Build history of the part. All positions in model axes, mm. Give positions to 0.01 mm unless a question says otherwise; leave off trailing zeros. Order: outer loops, then holes, each group sorted by start corner. A loop starts at its lowest first (then second) coordinate and runs counter-clockwise, first axis right, second up. Notation, with made-up numbers: (33.5, -39.75) - (59.5, -39.75) arc R21 ccw to (59.5, -26.75) - close; hole circle Ø6 at (-20, 63.25). An arc over 180 degrees is marked (long way). Answer in a Markdown table with one row per item.
```python
from build123d import *

# Parameters (mm, degrees)
F0_R     = 1.25
F0_R_2   = 5.5
F1_DEPTH = 4
F3_DEPTH = 2
F4_SIZE  = 2


# Not quite as in the source:
# - a feature names something its author has since deleted; it is built from what else it names


with BuildPart() as f1:
    # F0 (on Top) → F1 (new body)
    with BuildSketch(Plane.XY):
        with BuildLine():
            ThreePointArc((-36.0336562554, 5.4360876058), (-41.0336562554, 10.4360876058), (-46.0336562554, 5.4360876058))
            ThreePointArc((-46.0336562554, 5.4360876058), (-48.7113140605, 0.9910484741), (-53.6336562554, -0.6517453414))
            Line((-53.6336562554, -0.6517453414), (-57.6336562554, -0.6517453414))
            Line((-57.6336562554, -0.6517453414), (-59.4336562554, -0.6517453414))
            Line((-59.4336562554, -0.6517453414), (-59.4336562554, -1.3484233022))
            ThreePointArc((-59.4336562554, -1.3484233022), (-52.8307134237, -18.2761605269), (-36.5097932518, -26.2620672584))
            Line((-36.5097932518, -26.2620672584), (33.4902067482, -32.0954005917))
            ThreePointArc((33.4902067482, -32.0954005917), (52.4940809692, -25.5788138039), (60.5663437446, -7.1817566356))
            Line((60.5663437446, -7.1817566356), (60.5663437446, 8.4782659528))
            ThreePointArc((60.5663437446, 8.4782659528), (52.4940809692, 26.8753231211), (33.4902067482, 33.3919099089))
            Line((33.4902067482, 33.3919099089), (-36.5097932518, 27.5585765756))
            ThreePointArc((-36.5097932518, 27.5585765756), (-52.8307134237, 19.5726698441), (-59.4336562554, 2.6449326195))
            Line((-59.4336562554, 2.6449326195), (-59.4336562554, 1.9482546586))
            Line((-59.4336562554, 1.9482546586), (-57.6336562554, 1.9482546586))
            Line((-57.6336562554, 1.9482546586), (-53.6336562554, 1.9482546586))
            ThreePointArc((-53.6336562554, 1.9482546586), (-50.3543429782, 2.8450290737), (-48.4065189788, 5.6314392355))
            ThreePointArc((-48.4065189788, 5.6314392355), (-40.8279863477, 12.5929298404), (-33.4336562554, 5.4360876058))
            ThreePointArc((-33.4336562554, 5.4360876058), (-31.5267024615, 2.8420068396), (-28.4336562554, 1.9482546586))
            Line((-28.4336562554, 1.9482546586), (-15.4336562554, 1.9482546586))
            Line((-15.4336562554, 1.9482546586), (-15.4336562554, 15.2482546586))
            Line((-15.4336562554, 15.2482546586), (-4.9336562554, 15.2482546586))
            Line((-4.9336562554, 15.2482546586), (-4.9336562554, 17.1757546586))
            ThreePointArc((-4.9336562554, 17.1757546586), (-0.8336562554, 21.2757546586), (3.2663437446, 17.1757546586))
            Line((3.2663437446, 17.1757546586), (3.2663437446, 15.2482546586))
            Line((3.2663437446, 15.2482546586), (29.2163437446, 15.2482546586))
            Line((29.2163437446, 15.2482546586), (29.2163437446, 17.1757546586))
            ThreePointArc((29.2163437446, 17.1757546586), (33.3163437446, 21.2757546586), (37.4163437446, 17.1757546586))
            Line((37.4163437446, 17.1757546586), (37.4163437446, 15.2482546586))
            Line((37.4163437446, 15.2482546586), (47.9163437446, 15.2482546586))
            Line((47.9163437446, 15.2482546586), (47.9163437446, -13.9517453414))
            Line((47.9163437446, -13.9517453414), (37.4163437446, -13.9517453414))
            Line((37.4163437446, -13.9517453414), (37.4163437446, -15.8792453414))
            ThreePointArc((37.4163437446, -15.8792453414), (33.3163437446, -19.9792453414), (29.2163437446, -15.8792453414))
            Line((29.2163437446, -15.8792453414), (29.2163437446, -13.9517453414))
            Line((29.2163437446, -13.9517453414), (3.2663437446, -13.9517453414))
            Line((3.2663437446, -13.9517453414), (3.2663437446, -15.8792453414))
            ThreePointArc((3.2663437446, -15.8792453414), (-0.8336562554, -19.9792453414), (-4.9336562554, -15.8792453414))
            Line((-4.9336562554, -15.8792453414), (-4.9336562554, -13.9517453414))
            Line((-4.9336562554, -13.9517453414), (-15.4336562554, -13.9517453414))
            Line((-15.4336562554, -13.9517453414), (-15.4336562554, -0.6517453414))
            Line((-15.4336562554, -0.6517453414), (-28.4336562554, -0.6517453414))
            ThreePointArc((-28.4336562554, -0.6517453414), (-33.3559984503, 0.991048474), (-36.0336562554, 5.4360876058))
        make_face()
        with Locations((-34.4336562554, -13.8484233022)):
            Circle(F0_R, mode=Mode.SUBTRACT)
        with Locations((33.4902067482, -25.3792453414)):
            Circle(F0_R, mode=Mode.SUBTRACT)
        with Locations((-34.4336562554, 15.1449326195)):
            Circle(F0_R, mode=Mode.SUBTRACT)
        with Locations((33.4321971192, 26.6757546586)):
            Circle(F0_R, mode=Mode.SUBTRACT)
        with BuildLine():
            ThreePointArc((-53.6336562554, -0.6517453414), (-48.7113140605, 0.9910484741), (-46.0336562554, 5.4360876058))
            ThreePointArc((-46.0336562554, 5.4360876058), (-41.0336562554, 10.4360876058), (-36.0336562554, 5.4360876058))
            ThreePointArc((-36.0336562554, 5.4360876058), (-33.3559984503, 0.991048474), (-28.4336562554, -0.6517453414))
            Line((-28.4336562554, -0.6517453414), (-15.4336562554, -0.6517453414))
            Line((-15.4336562554, -0.6517453414), (-15.4336562554, -13.9517453414))
            Line((-15.4336562554, -13.9517453414), (-4.9336562554, -13.9517453414))
            Line((-4.9336562554, -13.9517453414), (-4.9336562554, -15.8792453414))
            ThreePointArc((-4.9336562554, -15.8792453414), (-0.8336562554, -19.9792453414), (3.2663437446, -15.8792453414))
            Line((3.2663437446, -15.8792453414), (3.2663437446, -13.9517453414))
            Line((3.2663437446, -13.9517453414), (29.2163437446, -13.9517453414))
            Line((29.2163437446, -13.9517453414), (29.2163437446, -15.8792453414))
            ThreePointArc((29.2163437446, -15.8792453414), (33.3163437446, -19.9792453414), (37.4163437446, -15.8792453414))
            Line((37.4163437446, -15.8792453414), (37.4163437446, -13.9517453414))
            Line((37.4163437446, -13.9517453414), (47.9163437446, -13.9517453414))
            Line((47.9163437446, -13.9517453414), (47.9163437446, 15.2482546586))
            Line((47.9163437446, 15.2482546586), (37.4163437446, 15.2482546586))
            Line((37.4163437446, 15.2482546586), (37.4163437446, 17.1757546586))
            ThreePointArc((37.4163437446, 17.1757546586), (33.3163437446, 21.2757546586), (29.2163437446, 17.1757546586))
            Line((29.2163437446, 17.1757546586), (29.2163437446, 15.2482546586))
            Line((29.2163437446, 15.2482546586), (3.2663437446, 15.2482546586))
            Line((3.2663437446, 15.2482546586), (3.2663437446, 17.1757546586))
            ThreePointArc((3.2663437446, 17.1757546586), (-0.8336562554, 21.2757546586), (-4.9336562554, 17.1757546586))
            Line((-4.9336562554, 17.1757546586), (-4.9336562554, 15.2482546586))
            Line((-4.9336562554, 15.2482546586), (-15.4336562554, 15.2482546586))
            Line((-15.4336562554, 15.2482546586), (-15.4336562554, 1.9482546586))
            Line((-15.4336562554, 1.9482546586), (-28.4336562554, 1.9482546586))
            ThreePointArc((-28.4336562554, 1.9482546586), (-31.5267024615, 2.8420068396), (-33.4336562554, 5.4360876058))
            ThreePointArc((-33.4336562554, 5.4360876058), (-40.8279863477, 12.5929298404), (-48.4065189788, 5.6314392355))
            ThreePointArc((-48.4065189788, 5.6314392355), (-50.3543429782, 2.8450290737), (-53.6336562554, 1.9482546586))
            Line((-53.6336562554, 1.9482546586), (-53.6336562554, -0.6517453414))
        make_face()
        with Locations((-4.4336562554, 0.6572546586)):
            Circle(F0_R_2, mode=Mode.SUBTRACT)
        Polygon((-59.4336562554, -0.6517453414), (-57.6336562554, -0.6517453414), (-57.6336562554, 0.6482546586), (-57.6336562554, 1.9482546586), (-59.4336562554, 1.9482546586), align=None)
        Polygon((-57.6336562554, -0.6517453414), (-53.6336562554, -0.6517453414), (-53.6336562554, 1.9482546586), (-57.6336562554, 1.9482546586), (-57.6336562554, 0.6482546586), align=None)
    extrude(amount=F1_DEPTH)

    # F2 (on face) → F3 (join)
    with BuildSketch(Plane(origin=(0, 0, 0), x_dir=(1, 0, 0), z_dir=(0, 0, -1))):
        with BuildLine():
            ThreePointArc((-53.8336562554, -1.7482546586), (-53.6922348992, -1.6896760149), (-53.6336562554, -1.5482546586))
            Line((-53.6336562554, -1.5482546586), (-53.6336562554, 0.2517453414))
            ThreePointArc((-53.6336562554, 0.2517453414), (-53.6922348992, 0.3931666976), (-53.8336562554, 0.4517453414))
            Line((-53.8336562554, 0.4517453414), (-57.4336562554, 0.4517453414))
            ThreePointArc((-57.4336562554, 0.4517453414), (-57.5750776116, 0.3931666976), (-57.6336562554, 0.2517453414))
            Line((-57.6336562554, 0.2517453414), (-57.6336562554, -0.6482546586))
            Line((-57.6336562554, -0.6482546586), (-57.6336562554, -1.5482546586))
            ThreePointArc((-57.6336562554, -1.5482546586), (-57.5750776116, -1.6896760149), (-57.4336562554, -1.7482546586))
            Line((-57.4336562554, -1.7482546586), (-53.8336562554, -1.7482546586))
        make_face()
    extrude(amount=F3_DEPTH)

    # F4
    f4_edges = [f1.edges().sort_by_distance(p)[0] for p in [
        (-35.683656, 15.144933, 4),
        (-35.683656, -13.848423, 4),
        (32.182197, 26.675755, 4),
        (32.240207, -25.379245, 4),
    ]]
    chamfer(f4_edges, length=F4_SIZE)


solid = f1.part
```
1. Cut at D-D on x = -34.5. Count the separate pieces of the cut face and the enclosed holes in it, and give its area (3 significant figures).
Check result:
| item | result |
|---|---|
| separate pieces | 3 |
| enclosed holes | 0 |
| area | 189 mm² |
2. Cut at A-A on x = -5.5. Write the cut outline in (y, z).
Check result:
| item | result |
|---|---|
| outline | (-28.85, 0) - (-4.74, 0) - (-4.74, 4) - (-28.85, 4) - close; (6.05, 0) - (30.14, 0) - (30.14, 4) - (6.05, 4) - close |
3. Cut at B-B on z = 1.1. Write the cut outline in (x, y), and give its area (3 significant figures).
Check result:
| item | result |
|---|---|
| outline | (-59.43, -1.35) arc R25 ccw to (-36.51, -26.26) - (33.49, -32.1) arc R25 ccw to (60.57, -7.18) - (60.57, 8.48) arc R25 ccw to (33.49, 33.39) - (-36.51, 27.56) arc R25 ccw to (-59.43, 2.64) - close; hole circle Ø2.5 at (-34.43, -13.85); hole circle Ø2.5 at (-34.43, 15.14); hole circle Ø11 at (-4.43, 0.66); hole circle Ø2.5 at (33.43, 26.68); hole circle Ø2.5 at (33.49, -25.38) |
| area | 6,540 mm² |
4. Drop flat-ended pins along their axis: P1, Ø2, axis at x = -29.5, y = -0.5, coming from the -Z side; P2, Ø0.6, axis at x = -55, z = -1, coming from the +Y side; P3, Ø4, axis at x = 33.43, y = 26.68, coming from the +Z side. Give the stop position or say it passes through.
Check result:
| item | result |
|---|---|
| P1 | stops at z = 0 |
| P2 | stops at y = 1.75 |
| P3 | stops at z = 2.75 |
5. Cut at C-C on y = 4.5. Write the cut outline in (x, z), and give its area (3 significant figures).
Check result:
| item | result |
|---|---|
| outline | (-59.36, 0) - (-8.37, 0) - (-8.37, 4) - (-59.36, 4) - close; (-0.5, 0) - (60.57, 0) - (60.57, 4) - (-0.5, 4) - close |
| area | 448 mm² |
6. Probe line 1 (Z direction, x = -1, y = -17.5); line 2 (X direction, y = -13, z = 3.3); line 3 (X direction, y = 14, z = 2.3). List the from-to ranges inside material, lowest first.
Check result:
| item | result |
|---|---|
| line 1 | z = 0 to 4 |
| line 2 | x = -56.55 to -36.84, -32.03 to 59.88 |
| line 3 | x = -56.71 to -35.48, -33.39 to 59.95 |
7. Two-plate mould, pull along X, no slides. Class faces 1 (the face through (32.183, 26.731, 0.986)), 2 (the face through (0, -6, 0)), 3 (the face through (-52.653, 19.763, 1.972)): +X half, -X half, draft (parallel to the pull), parting line (faces both ways), or undercut.
Check result:
| item | result |
|---|---|
| face 1 | undercut |
| face 2 | draft |
| face 3 | -X half |
